Build history of the part. All positions in model axes, mm. Face numbers are marked on the shaded views. A direction names the side the tool comes from. Give positions to 0.01 mm unless a question says otherwise; leave off trailing zeros. Write each loop counter-clockwise with the first axis right and the second up, starting at its lowest first coordinate (ties: lowest second). Pieces come first, ordered by that corner, then holes.
Autodesk Inventor part; units mm, degrees
ref_plane "YZ Plane" through (0, 0, 0) normal (1, 0, 0) x (0, 1, 0)
ref_plane "XZ Plane" through (0, 0, 0) normal (0, 1, 0) x (-1, 0, 0)
ref_plane "XY Plane" through (0, 0, 0) normal (0, 0, 1) x (1, 0, 0)
sketch "Sketch1" plane through (0, 0, 0) normal (0, 0, 1) x (1, 0, 0)
  line L0 (-10, -6) -> (10, -6)
  line L1 (10, -6) -> (10, 6)
  line L2 (10, 6) -> (-10, 6)
  line L3 (-10, 6) -> (-10, -6)
  circle A0 centre (-6, 2.5) radius 1.6
  circle A1 centre (6, 2.5) radius 1.6
  line L4 (-10, -6) -> (10, -6)
  line L5 (10, -6) -> (10, -3)
  line L6 (10, -3) -> (-10, -3)
  line L7 (-10, -3) -> (-10, -6)
  point P0 (0, 0)
  point P1 (0, 6)
  point P2 (-10, 0)
  dimension "d0" = 12
  dimension "d1" = 20
  dimension "d2" = 3.2
  dimension "d3" = 3.2
  dimension "d4" = 12
  dimension "d5" = 6
  dimension "d6" = 2.5
  dimension "d7" = 3
extrude "Extrusion1" add sketch "Sketch1" along normal blind 3 contours L3 L2 L1 L6
extrude "Extrusion2" add sketch "Sketch1" along normal blind 18 contours L3 L6 L1 L0
sketch "Sketch2" plane through (-10, -6, 0) normal (0, -1, 0) x (1, 0, 0)
  line L0 (20, 0) -> (0, 0)
  line L1 (0, 0) -> (0, 18)
  line L2 (0, 18) -> (20, 18)
  line L3 (20, 18) -> (20, 0)
  circle A0 centre (5.25, 14.5) radius 1.35
  circle A1 centre (14.75, 14.5) radius 1.35
  point P0 (10, 0)
  dimension "d13" = 9.5
  dimension "d14" = 5.25
  dimension "d15" = 2.7
  dimension "d16" = 2.7
  dimension "d17" = 3.5
extrude "Extrusion3" cut sketch "Sketch2" against normal up to surface (3 mm away) contours A0 | A1
chamfer "Chamfer1" distance 1 angle 45 2 edges at (10, 6, 1.5) (-10, 6, 1.5)
properties part number "LimitSwitch_TopHolder"
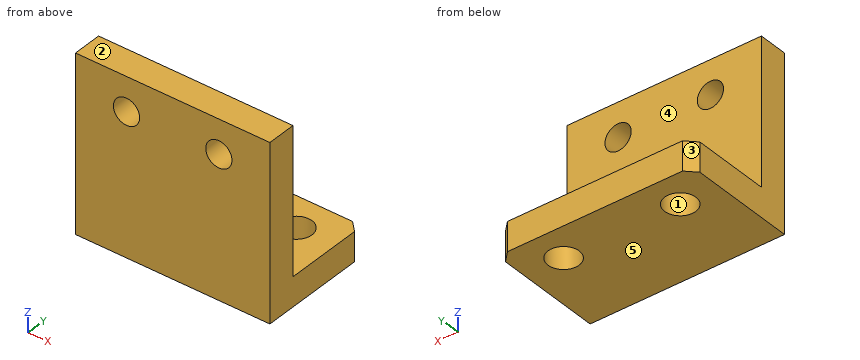
(1) Drop flat-ended pins along their axis: pin 1 (3 mm diameter, centred on x = -5.5, z = 15.5, fed in from +Y); pin 2 (4 mm diameter, centred on x = 4, y = -4.5, fed in from -Z); pin 3 (2.5 mm diameter, centred on x = -0.5, y = 1.5, fed in from +Z). Give the stop position or say it passes through.
(2) Saw through at B-B, the plane y = 2.5. List the corners of the cut face in (x, z).
(3) Probe line 1 (Y direction, x = -6, z = 1.15); line 2 (Z direction, x = -4.75, y = -5.3); line 3 (Z direction, x = 8.25, y = 5.75). List the from-to ranges inside material, lowest first.
(4) 3-axis set-ups, long thin cutter, end or side, ignore diameter. For the marked faces 4 and 5: which of +Z, -Z, +X, -X, +Y, -Y reach the whole face in a straight line?
(5) Saw through at A-A, the plane z = 14.5. List the corners of the cut face in (x, y).
(6) Mould opens along Y. For the marked faces 1, 2 and 3 say: +Y half, -Y half, draft (parallel to the pull), parting line (faces both ways), or undercut.
(7) Saw through at D-D, the plane x = -4.75. List the corners of the cut face in (y, z).
(8) Saw through at C-C, the plane y = -5. List the corners of the cut face in (x, z), plus the area to 3 significant figures.
Computed values:
1. pin 1: stops at y = -3
1. pin 2: stops at z = 0
1. pin 3: stops at z = 3
2. outline: (-10, 0) - (-7.6, 0) - (-7.6, 3) - (-10, 3) - close; (-4.4, 0) - (4.4, 0) - (4.4, 3) - (-4.4, 3) - close; (7.6, 0) - (10, 0) - (10, 3) - (7.6, 3) - close
3. line 1: y = -6 to 0.9, 4.1 to 6
3. line 2: z = 0 to 13.15, 15.85 to 18
3. line 3: z = 0 to 3
4. face 4: +Z, +X, -X, +Y
4. face 5: -Z, +X, -X, +Y, -Y
5. outline: (-10, -6) - (-6.1, -6) - (-6.1, -3) - (-10, -3) - close; (-3.4, -6) - (3.4, -6) - (3.4, -3) - (-3.4, -3) - close; (6.1, -6) - (10, -6) - (10, -3) - (6.1, -3) - close
6. face 1: undercut
6. face 2: draft
6. face 3: +Y half
7. outline: (-6, 0) - (1.5, 0) - (1.5, 3) - (-3, 3) - (-3, 13.15) - (-6, 13.15) - close; (-6, 15.85) - (-3, 15.85) - (-3, 18) - (-6, 18) - close; (3.5, 0) - (6, 0) - (6, 3) - (3.5, 3) - close
8. outline: (-10, 0) - (10, 0) - (10, 18) - (-10, 18) - close; hole circle Ø2.7 at (-4.75, 14.5); hole circle Ø2.7 at (4.75, 14.5)
8. area: 349 mm2
